The model under review builds one solid part; all positions refer to its coordinate system, in mm. Face numbers are marked on the shaded views. A direction names the side the tool comes from. Give positions to 0.01 mm unless a question says otherwise; leave off trailing zeros. Use CSV: the item, a comma, the result in double quotes. Start each with the question number.
1. Machinability: for the marked faces 1 and 2, which of the approach directions +Z, -Z, +X, -X, +Y, -Y give a long, thin tool a straight path to every point of the face, cutting with its end or side? Answer none if there is none.
2. For pin 1 (1.5 mm diameter, centred on x = 121, y = -6, fed in from -Z); pin 2 (3.5 mm diameter, centred on x = 30, y = -7, fed in from -Z); pin 3 (4 mm diameter, centred on x = 88, y = 0, fed in from +Z); pin 4 (6.5 mm diameter, centred on x = 58, y = 7, fed in from +Z), all flat-tipped, find the tip position at first contact; note any pin that passes through.
3. To check wall thickness, follow line 1 (Y direction, x = 58, z = 29.3); line 2 (Y direction, x = 121, z = 25.6); line 3 (X direction, y = 6, z = 26.55). State the ranges of each line that lie inside material, in increasing order. Write a range as [from, to].
```python
from build123d import *

# Parameters (mm, degrees)
EXTRUDE_1_DEPTH     = 5
SKETCH_1_3_R        = 1.1
CUT_EXTRUDE_2_DEPTH = 187.33571853
SKETCH_1_4_R        = 2.55
CUT_EXTRUDE_3_DEPTH = 2.6
SKETCH_2_R          = 1.25
CUT_EXTRUDE_4_DEPTH = 187.33571853
CUT_EXTRUDE_START   = -5
SKETCH_2_3_R        = 2
CUT_EXTRUDE_5_DEPTH = 2.5
SKETCH_3_W          = 59
SKETCH_3_H          = 2.6
CUT_EXTRUDE_6_DEPTH = 188.138985783
CUT_EXTRUDE_7_DEPTH = 187.33571853
SKETCH_5_W          = 276.925102881
SKETCH_5_H          = 124.694650206
CUT_EXTRUDE_8_DEPTH = 187.871613682


with BuildPart() as part:
    # 草图1 → 凸台-拉伸1 (new body)
    with BuildSketch(Plane.XY):
        with BuildLine():
            Line((0, -10), (176, -10))
            ThreePointArc((176, -10), (186, 0), (176, 10))
            Line((176, 10), (0, 10))
            ThreePointArc((0, 10), (-10, 0), (0, -10))
        make_face()
    extrude(amount=EXTRUDE_1_DEPTH)

    # 草图1<3> → 切除-拉伸2 (cut, through all)
    with BuildSketch(Plane.XY):
        with Locations((88, 0)):
            Circle(SKETCH_1_3_R)
        Circle(SKETCH_1_3_R)
    extrude(amount=CUT_EXTRUDE_2_DEPTH, mode=Mode.SUBTRACT)

    # 草图1<4> → 切除-拉伸3 (cut)
    with BuildSketch(Plane.XY):
        with Locations((88, 0)):
            Circle(SKETCH_1_4_R)
        Circle(SKETCH_1_4_R)
    extrude(amount=CUT_EXTRUDE_3_DEPTH, mode=Mode.SUBTRACT)

    # 草图2 → 切除-拉伸4 (cut, through all)
    with BuildSketch(Plane(origin=(0, 0, 0), x_dir=(-1, 0, 0), z_dir=(0, 0, -1))):
        with Locations((-121, -6)):
            Circle(SKETCH_2_R)
        with Locations((-121, 6)):
            Circle(SKETCH_2_R)
        with Locations((-114, 0)):
            Circle(SKETCH_2_R)
        with Locations((-58, 7)):
            Circle(SKETCH_2_R)
        with Locations((-30, 7)):
            Circle(SKETCH_2_R)
        with Locations((-58, -7)):
            Circle(SKETCH_2_R)
        with Locations((-30, -7)):
            Circle(SKETCH_2_R)
    extrude(amount=-CUT_EXTRUDE_4_DEPTH, mode=Mode.SUBTRACT)

    # 草图2<3> → 切除-拉伸5 (cut)
    with BuildSketch(Plane(origin=(0, 0, 0), x_dir=(-1, 0, 0), z_dir=(0, 0, -1)).offset(CUT_EXTRUDE_START)):
        with Locations(Location((-121, -6, 0), (0, 0, 180))):
            Circle(SKETCH_2_3_R)
        with Locations(Location((-121, 6, 0), (0, 0, 180))):
            Circle(SKETCH_2_3_R)
        with Locations(Location((-114, 0, 0), (0, 0, 180))):
            Circle(SKETCH_2_3_R)
        with Locations(Location((-58, 7, 0), (0, 0, 180))):
            Circle(SKETCH_2_3_R)
        with Locations(Location((-30, 7, 0), (0, 0, 180))):
            Circle(SKETCH_2_3_R)
        with Locations(Location((-58, -7, 0), (0, 0, 180))):
            Circle(SKETCH_2_3_R)
        with Locations(Location((-30, -7, 0), (0, 0, 180))):
            Circle(SKETCH_2_3_R)
    extrude(amount=CUT_EXTRUDE_5_DEPTH, mode=Mode.SUBTRACT)

    # 草图3 → 切除-拉伸6 (cut, through all)
    with BuildSketch(Plane(origin=(0, 10, 0), x_dir=(1, 0, 0), z_dir=(0, 1, 0))):
        with Locations((156.5, -1.3)):
            Rectangle(SKETCH_3_W, SKETCH_3_H)
    extrude(amount=-CUT_EXTRUDE_6_DEPTH, mode=Mode.SUBTRACT)

    # 草图4 → 切除-拉伸7 (cut, through all)
    with BuildSketch(Plane.XY.offset(5)):
        with BuildLine():
            Line((164.2, -2.4), (154, -2.4))
            ThreePointArc((154, -2.4), (152.4, -4), (154, -5.6))
            Line((154, -5.6), (164.2, -5.6))
            ThreePointArc((164.2, -5.6), (165.8, -4), (164.2, -2.4))
        make_face()
        with BuildLine():
            ThreePointArc((154, 5.6), (152.4, 4), (154, 2.4))
            Line((154, 2.4), (164.2, 2.4))
            ThreePointArc((164.2, 2.4), (165.8, 4), (164.2, 5.6))
            Line((164.2, 5.6), (154, 5.6))
        make_face()
    extrude(amount=-CUT_EXTRUDE_7_DEPTH, mode=Mode.SUBTRACT)


with BuildPart() as body_2:
    # 镜向2: mirrored copy
    add(part.part.mirror(Plane.XY.offset(15)))


with BuildPart() as part_1:
    add(part.part)

    # 草图5 → 切除-拉伸8 (cut, through all)
    with BuildSketch(Plane.XY.offset(15)):
        with Locations((84.530041153, -5.708641975)):
            Rectangle(SKETCH_5_W, SKETCH_5_H)
    extrude(amount=-CUT_EXTRUDE_8_DEPTH, mode=Mode.SUBTRACT)


solid = body_2.part
```
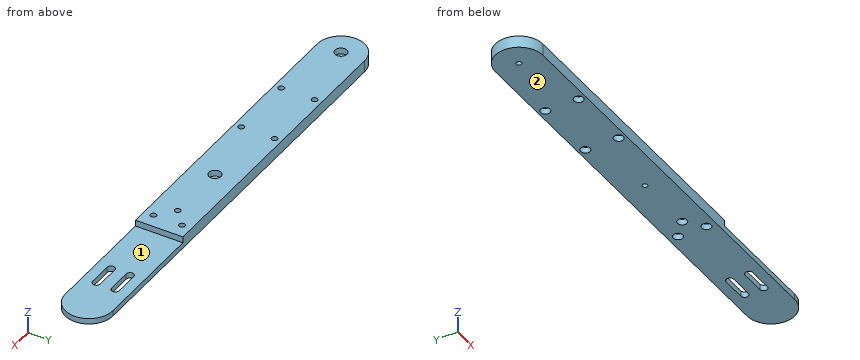
Determined:
1,face 1,"+Z, +X, +Y, -Y"
1,face 2,"-Z, +X, -X, +Y, -Y"
2,pin 1,"passes through"
2,pin 2,"stops at z = 27.5"
2,pin 3,"stops at z = 27.4"
2,pin 4,"stops at z = 30"
3,line 1,"y = [-10, -8.25], [-5.75, 5.75], [8.25, 10]"
3,line 2,"y = [-10, -8], [-4, 4], [8, 10]"
3,line 3,"x = [-8, 28.27], [31.73, 56.27], [59.73, 119], [123, 184]"
